Verification items for the finished model (mm, model axes). Give positions to 0.01 mm unless a question says otherwise; leave off trailing zeros. Loops run counter-clockwise (first coordinate to the right, second up) from the corner with the lowest first, then second, coordinate; pieces in that order, holes last. Notation, with made-up numbers: M 87.25,-3 L 126.25,-3 A9 cw 126.25,11 Z; hole C 86.25,64.5 d6. An arc over 180 degrees is marked long. Answer in a Markdown table with one row per item.
```python
from build123d import *

# Parameters (mm, degrees)
ESQUISSE1_W             = 30
ESQUISSE1_H             = 20
BOSS_EXTRU_1_DEPTH      = 130
ESQUISSE2_R             = 1.65
ENL_V_MAT_EXTRU_1_DEPTH = 135.907375632
ESQUISSE3_R             = 1.65
ENL_V_MAT_EXTRU_2_DEPTH = 135.907375632


with BuildPart() as part:
    # Esquisse1 → Boss.-Extru.1 (new body)
    with BuildSketch(Plane.XY):
        with Locations((15, 10)):
            Rectangle(ESQUISSE1_W, ESQUISSE1_H)
    extrude(amount=BOSS_EXTRU_1_DEPTH)

    # Esquisse2 → Enlèv. mat.-Extru.1 (cut, through all)
    with BuildSketch(Plane(origin=(0, 20, 0), x_dir=(1, 0, 0), z_dir=(0, 1, 0))):
        with Locations(Location((5, -117.5, 0), (0, 0, 270))):
            Circle(ESQUISSE2_R)
        with Locations(Location((5, -102.5, 0), (0, 0, 90))):
            Circle(ESQUISSE2_R)
        with Locations(Location((25, -102.5, 0), (0, 0, 270))):
            Circle(ESQUISSE2_R)
        with Locations(Location((25, -117.5, 0), (0, 0, 90))):
            Circle(ESQUISSE2_R)
        with Locations(Location((25, -12.5, 0), (0, 0, 270))):
            Circle(ESQUISSE2_R)
        with Locations(Location((25, -27.5, 0), (0, 0, 90))):
            Circle(ESQUISSE2_R)
        with Locations(Location((5, -27.5, 0), (0, 0, 270))):
            Circle(ESQUISSE2_R)
        with Locations(Location((5, -12.5, 0), (0, 0, 90))):
            Circle(ESQUISSE2_R)
    extrude(amount=-ENL_V_MAT_EXTRU_1_DEPTH, mode=Mode.SUBTRACT)

    # Esquisse3 → Enlèv. mat.-Extru.2 (cut, through all)
    with BuildSketch(Plane(origin=(30, 0, 0), x_dir=(0, 0, -1), z_dir=(1, 0, 0))):
        with Locations((-65, 10)):
            Circle(ESQUISSE3_R)
        with Locations((-95, 10)):
            Circle(ESQUISSE3_R)
        with Locations((-125, 10)):
            Circle(ESQUISSE3_R)
        with Locations(Location((-5, 10, 0), (0, 0, 180))):
            Circle(ESQUISSE3_R)
        with Locations(Location((-35, 10, 0), (0, 0, 180))):
            Circle(ESQUISSE3_R)
    extrude(amount=-ENL_V_MAT_EXTRU_2_DEPTH, mode=Mode.SUBTRACT)


solid = part.part
```
Item 1: Sectioned sample at D-D (x = 10.75). Record the cut outline in (y, z).
Reported:
| item | result |
|---|---|
| outline | M 0,0 L 20,0 L 20,130 L 0,130 Z; hole C 10,5 d3.3; hole C 10,35 d3.3; hole C 10,65 d3.3; hole C 10,95 d3.3; hole C 10,125 d3.3 |
Item 2: Release check for a two-part mould opening along X. For faces 1 (the cylindrical face through (15.21, 10.07, 66.65)), 2 (the flat face through (30, 12, 64)), 3 (the cylindrical face through (5.632, 10.14, 10.976)), 4 (the flat face through (0, 12, 64)) record: released by +X, released by -X, zero draft, split by the parting line, or undercut.
Reported:
| item | result |
|---|---|
| face 1 | zero draft |
| face 2 | released by +X |
| face 3 | undercut |
| face 4 | released by -X |
Item 3: Sectioned sample at A-A (y = 10). State how many separate pieces and enclosed holes the cut face has, and give its area (3 significant figures).
Reported:
| item | result |
|---|---|
| separate pieces | 6 |
| enclosed holes | 8 |
| area | 3,340 mm^2 |
Item 4: Scan lines: L1, parallel to X at y = 14.25, z = 12.5; L2, parallel to Z at x = 8.25, y = 10.5; L3, parallel to Y at x = 23.5, z = 125. Record each from-to range of solid material in increasing order. Write a range as [from, to].
Reported:
| item | result |
|---|---|
| L1 | x = [0, 3.35], [6.65, 23.35], [26.65, 30] |
| L2 | z = [0, 3.43], [6.57, 33.43], [36.57, 63.43], [66.57, 93.43], [96.57, 123.43], [126.57, 130] |
| L3 | y = [0, 8.35], [11.65, 20] |
Item 5: Sectioned sample at C-C (z = 117.5). Record the cut outline in (x, y), and give its area (3 significant figures).
Reported:
| item | result |
|---|---|
| outline | M 0,0 L 3.35,0 L 3.35,20 L 0,20 Z; M 6.65,0 L 23.35,0 L 23.35,20 L 6.65,20 Z; M 26.65,0 L 30,0 L 30,20 L 26.65,20 Z |
| area | 468 mm^2 |
Item 6: Go/stop test with flat-tipped pins: pin 1 (10 mm diameter, centred on x = 9, y = 9, fed in from -Z); pin 2 (2 mm diameter, centred on x = 25, z = 117.5, fed in from -Y). Record where each tip stops, or that it passes through.
Reported:
| item | result |
|---|---|
| pin 1 | stops at z = 0 |
| pin 2 | passes through |
